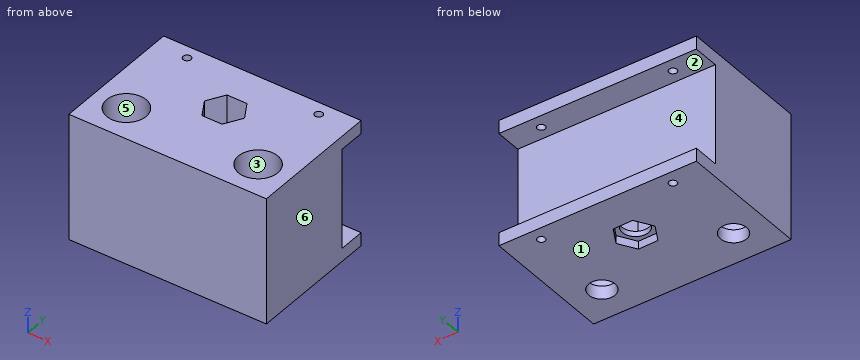
Autodesk Inventor part; units mm, degrees
ref_plane "YZ Plane" through (0, 0, 0) normal (1, 0, 0) x (0, 1, 0)
ref_plane "XZ Plane" through (0, 0, 0) normal (0, 1, 0) x (-1, 0, 0)
ref_plane "XY Plane" through (0, 0, 0) normal (0, 0, 1) x (1, 0, 0)
sketch "Sketch11" plane through (0, 0, 0) normal (0, 0, 1) x (1, 0, 0)
  line L0 (3.7722, 0) -> (78.7722, 0)
  line L1 (78.7722, 0) -> (78.7722, 45)
  line L2 (78.7722, 45) -> (3.7722, 45)
  line L3 (3.7722, 45) -> (3.7722, 0)
  circle A0 centre (16.2722, 8) radius 5
  circle A1 centre (66.2722, 8) radius 5
  point P0 (0, 0)
  dimension "d63" = 75
  dimension "d65" = 45
  dimension "d66" = 10
  dimension "d67" = 10
  dimension "d68" = 50
  dimension "d69" = 12.5
  dimension "d70" = 8
  dimension "d71" = 8
extrude "Extrusion10" add sketch "Sketch11" along normal blind 5
sketch "Sketch12" plane through (0, 0, 5) normal (0, 0, 1) x (1, 0, 0)
  circle A0 centre (66.2722, 8) radius 5
  circle A1 centre (16.2722, 8) radius 5
  circle A2 centre (16.2722, 8) radius 7.5
  circle A3 centre (66.2722, 8) radius 7.5
  point P0 (0, 0)
  dimension "d74" = 15
  dimension "d77" = 15
sketch "Sketch13" plane through (0, 0, 5) normal (0, 0, 1) x (1, 0, 0)
  line L0 (3.7722, 0) -> (78.7722, 0)
  line L1 (3.7722, 45) -> (3.7722, 0)
  line L2 (37.4644, 31.6016) -> (45.0855, 31.5984)
  line L3 (45.0855, 31.5984) -> (48.8932, 24.9968)
  line L4 (48.8932, 24.9968) -> (45.0799, 18.3984)
  line L5 (45.0799, 18.3984) -> (37.4589, 18.4016)
  line L6 (37.4589, 18.4016) -> (33.6512, 25.0032)
  line L7 (33.6512, 25.0032) -> (37.4644, 31.6016)
  point P0 (0, 0)
  point P1 (41.2722, 25)
  point P2 (41.2722, 25)
  dimension "d81" = 37.5
  dimension "d82" = 25
  dimension "d83" = 13.2
sketch "Sketch14" plane through (0, 0, 5) normal (0, 0, 1) x (1, 0, 0)
  circle A0 centre (41.2722, 25) radius 5
  line L0 (3.7722, 0) -> (78.7722, 0)
  line L1 (3.7722, 45) -> (3.7722, 0)
  point P0 (0, 0)
  dimension "d87" = 10
  dimension "d89" = 25
  dimension "d90" = 37.5
extrude "Extrusion13" cut sketch "Sketch14" against normal blind 50
sketch "Sketch16" plane through (0, 0, 0) normal (0, 0, -1) x (-1, 0, 0)
  line L0 (-78.7722, 45) -> (-3.7722, 45)
  line L1 (-78.7722, 0) -> (-78.7722, 45)
  circle A0 centre (-66.2722, 40) radius 1.5
  circle A1 centre (-16.2722, 40) radius 1.5
  point P0 (0, 0)
  dimension "d99" = 3
  dimension "d101" = 3
  dimension "d102" = 5
  dimension "d103" = 5
  dimension "d104" = 50
  dimension "d105" = 12.5
extrude "Extrusion15" cut sketch "Sketch16" against normal blind 100
sketch "Sketch17" plane through (3.7722, 0, 0) normal (0, -1, 0) x (1, 0, 0)
  line L0 (0, 0) -> (75, 0)
  line L1 (75, 0) -> (75, 5)
  line L2 (0, 0) -> (75, 0)
  line L3 (75, 0) -> (75, 5)
  line L4 (75, 5) -> (0, 5)
  line L5 (0, 5) -> (0, 0)
  point P0 (-3.7722, 0)
extrude "Extrusion16" add sketch "Sketch17" along normal blind 5
sketch "Sketch20" plane through (0, 0, 0) normal (0, 0, -1) x (-1, 0, 0)
  circle A0 centre (-41.2722, 25) radius 5
  line L0 (-45.1434, 31.4302) -> (-37.6391, 31.5677)
  line L1 (-37.6391, 31.5677) -> (-33.7679, 25.1375)
  line L2 (-33.7679, 25.1375) -> (-37.401, 18.5698)
  line L3 (-37.401, 18.5698) -> (-44.9052, 18.4323)
  line L4 (-44.9052, 18.4323) -> (-48.7765, 24.8625)
  line L5 (-48.7765, 24.8625) -> (-45.1434, 31.4302)
  point P0 (0, 0)
  dimension "d122" = 13
extrude "Extrusion19" cut sketch "Sketch20" against normal blind 3
sketch "Sketch21" plane through (0, 0, 5) normal (0, 0, 1) x (1, 0, 0)
  circle A0 centre (41.2722, 25) radius 5
  circle A1 centre (66.2722, 8) radius 5
  circle A2 centre (16.2722, 8) radius 5
  line L0 (78.7722, 45) -> (78.7722, -5)
  line L1 (78.7722, 45) -> (3.7722, 45)
  line L2 (3.7722, -5) -> (78.7722, -5)
  line L3 (78.7722, -5) -> (78.7722, 35)
  line L4 (78.7722, 35) -> (3.7722, 35)
  line L5 (3.7722, 35) -> (3.7722, -5)
  point P0 (0, 0)
  dimension "d125" = 10
extrude "Extrusion20" add sketch "Sketch21" along normal blind 38
extrude "Extrusion22" cut sketch "Sketch12" along normal blind 38
extrude "Extrusion23" cut sketch "Sketch13" along normal blind 38
sketch "Sketch22" plane through (0, 0, 43) normal (0, 0, 1) x (1, 0, 0)
  line L0 (45.0855, 31.5984) -> (48.8932, 24.9968)
  line L1 (48.8932, 24.9968) -> (45.0799, 18.3984)
  line L2 (45.0799, 18.3984) -> (37.4589, 18.4016)
  line L3 (37.4589, 18.4016) -> (33.6512, 25.0032)
  line L4 (33.6512, 25.0032) -> (37.4644, 31.6016)
  line L5 (37.4644, 31.6016) -> (45.0855, 31.5984)
  circle A0 centre (16.2722, 8) radius 7.5
  circle A1 centre (66.2722, 8) radius 7.5
  line L6 (78.7722, 35) -> (3.7722, 35)
  line L7 (3.7722, -5) -> (78.7722, -5)
  line L8 (78.7722, -5) -> (78.7722, 45)
  line L9 (78.7722, 45) -> (3.7722, 45)
  line L10 (3.7722, 45) -> (3.7722, -5)
  point P0 (0, 0)
  dimension "d134" = 10
extrude "Extrusion24" add sketch "Sketch22" along normal blind 5
sketch "Sketch23" plane through (0, 0, 48) normal (0, 0, 1) x (1, 0, 0)
  line L0 (78.7722, 45) -> (3.7722, 45)
  line L1 (3.7722, 45) -> (3.7722, -5)
  circle A0 centre (16.2722, 40) radius 1.5
  circle A1 centre (66.2722, 40) radius 1.5
  point P0 (0, 0)
  dimension "d137" = 3
  dimension "d139" = 3
  dimension "d140" = 50
  dimension "d141" = 12.5
  dimension "d142" = 5
  dimension "d143" = 5
extrude "Extrusion25" cut sketch "Sketch23" against normal blind 5
properties part number "carriage"
Work out the finished part from the listing and answer in its coordinate system (mm). Face numbers are marked on the shaded views. A direction names the side the tool comes from. Round coordinates to 2 decimals unless told otherwise and drop trailing zeros. Write each loop counter-clockwise with the first axis right and the second up, starting at its lowest first coordinate (ties: lowest second). Pieces come first, ordered by that corner, then holes. Notation, with made-up numbers: (47, 87.25) -> (66, 87.25) arc R25 cw to (66, 110.25) -> close; hole circle Ø1 at (41, 6.25). An arc over 180 degrees is marked (long way). Write each question's results on one line, items separated by ' | '.
Item 1: Which of the six approach directions +Z, -Z, +X, -X, +Y, -Y give full straight-line access (tool end or side, diameter ignored) to the marked faces 1, 2 and 3?
Result set:
face 1: -Z, +X, -X, +Y, -Y | face 2: +X, -X, +Y | face 3: +Z
Item 2: A cutting plane is placed at A-A, the plane y = 40. Determine the outline of the cut face in (x, z).
Result set:
outline: (3.77, 0) -> (14.77, 0) -> (14.77, 5) -> (3.77, 5) -> close; (3.77, 43) -> (14.77, 43) -> (14.77, 48) -> (3.77, 48) -> close; (17.77, 0) -> (64.77, 0) -> (64.77, 5) -> (17.77, 5) -> close; (17.77, 43) -> (64.77, 43) -> (64.77, 48) -> (17.77, 48) -> close; (67.77, 0) -> (78.77, 0) -> (78.77, 5) -> (67.77, 5) -> close; (67.77, 43) -> (78.77, 43) -> (78.77, 48) -> (67.77, 48) -> close
Item 3: Find the intervals of material crossed by line 1 along Y through (x, z) = (45, 11); line 2 along Z through (x, y) = (59.5, 36); line 3 along Y through (x, z) = (50, 23.5), in increasing order. Write a range as [from, to].
Result set:
line 1: [-5, 18.4], [31.6, 35] | line 2: [0, 5], [43, 48] | line 3: [-5, 35]
Item 4: A cutting plane is placed at B-B, the plane z = 17. Determine the outline of the cut face in (x, y), plus the area to 3 significant figures.
Result set:
outline: (3.77, -5) -> (78.77, -5) -> (78.77, 35) -> (3.77, 35) -> close; hole circle Ø15 at (16.27, 8); hole (33.65, 25) -> (37.46, 18.4) -> (45.08, 18.4) -> (48.89, 25) -> (45.09, 31.6) -> (37.46, 31.6) -> close; hole circle Ø15 at (66.27, 8) | area: 2,500 mm^2
Item 5: Flat-ended cylindrical pins translate along their axes: P1, Ø13.5, axis at x = 66.27, y = 8, coming from the -Z side; P2, Ø6.5, axis at x = 43, y = 23, coming from the -Z side; P3, Ø4, axis at x = 43, z = 9, coming from the +Y side. Find the tip coordinate at first contact, or state that the pin passes through.
Result set:
P1: z = 0 | P2: z = 3 | P3: y = 35
Item 6: A cutting plane is placed at C-C, the plane y = 8. Determine the outline of the cut face in (x, z).
Result set:
outline: (3.77, 0) -> (11.27, 0) -> (11.27, 5) -> (8.77, 5) -> (8.77, 48) -> (3.77, 48) -> close; (21.27, 0) -> (61.27, 0) -> (61.27, 5) -> (58.77, 5) -> (58.77, 48) -> (23.77, 48) -> (23.77, 5) -> (21.27, 5) -> close; (71.27, 0) -> (78.77, 0) -> (78.77, 48) -> (73.77, 48) -> (73.77, 5) -> (71.27, 5) -> close
Item 7: A cutting plane is placed at D-D, the plane x = 40. Determine the outline of the cut face in (y, z), plus the area to 3 significant figures.
Result set:
outline: (-5, 0) -> (18.52, 0) -> (18.52, 3) -> (20.16, 3) -> (20.16, 5) -> (18.4, 5) -> (18.4, 48) -> (-5, 48) -> close; (29.84, 3) -> (31.52, 3) -> (31.52, 0) -> (45, 0) -> (45, 5) -> (35, 5) -> (35, 43) -> (45, 43) -> (45, 48) -> (31.6, 48) -> (31.6, 5) -> (29.84, 5) -> close | area: 1,390 mm^2
Item 8: The mould has two halves that part along X. Classify the marked faces 4, 5 and 6: +X half, -X half, draft (parallel to the pull), parting line (faces both ways), or undercut.
Result set:
face 4: draft | face 5: undercut | face 6: +X half
